Design review of the part built by this model. Coordinates are the model's own, in mm. Face numbers are marked on the shaded views. Coordinates: 2 decimals unless noted, no trailing zeros. Loops run counter-clockwise (first coordinate to the right, second up) from the corner with the lowest first, then second, coordinate; pieces in that order, holes last. Notation, with made-up numbers: (7, 64) - (58, 64) arc R35 cw to (58, 99) - close; hole circle Ø3 at (48, -7). An arc over 180 degrees is marked (long way). Use one line per item in the form item = value. Start each with the question number.
(1) For L1, parallel to Y at x = 4, z = 14; L2, parallel to X at y = 6.5, z = -1.5; L3, parallel to Z at x = 0, y = 16.75, list the stretches that pass through material, from the lowest coordinate up.
(2) Add section B-B (z = 0). State the section outline as (x, y) points.
(3) Clearance check with flat-ended pins moving along their axes: pin 1 Ø1.5 at (y, z) = (15.5, 0.5) entering from -X; pin 2 Ø10 at (x, y) = (2.5, 1) entering from +Z; pin 3 Ø8 at (x, y) = (-4.5, 1) entering from -Z; pin 4 Ø2 at (y, z) = (2, 8) entering from -X. State where each tip first meets the part, or that it passes through.
(4) The part is to be moulded in two halves that separate along X. For the marked faces 1, 2, 3 and 4, say which applies: pulls with the +X half, pulls with the -X half, needs draft (parallel to the pull), parting line crosses it, or undercut.
(5) Add section C-C (x = 6.5). State the section outline as (y, z) points, plus the area to 3 significant figures.
(6) Add section A-A (x = 0). State the section outline as (y, z) points, plus the area to 4 significant figures.
(7) Add section D-D (z = -12.5). State the section outline as (x, y) points, plus the area to 3 significant figures.
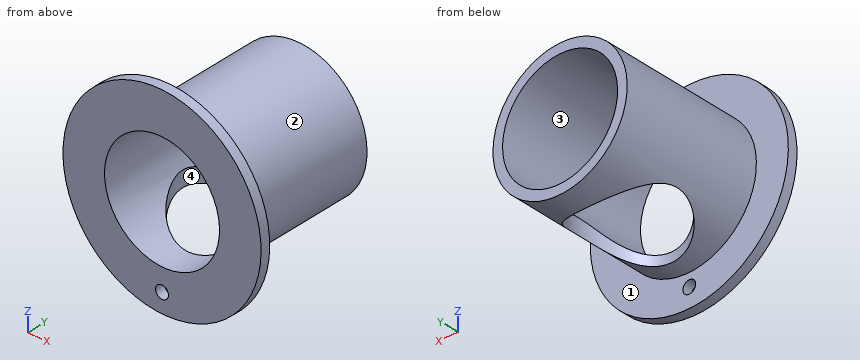
```python
from build123d import *

# Parameters (mm, degrees)
SKETCH1_R           = 10.5
SKETCH1_R_2         = 9
BOSS_EXTRUDE1_DEPTH = 38.3
SKETCH2_R           = 15.5
SKETCH2_R_2         = 9
SKETCH2_R_3         = 1
BOSS_EXTRUDE2_DEPTH = 1.5
SKETCH10_R          = 7.65
CUT_EXTRUDE1_DEPTH  = 46.437209421
SKETCH15_R          = 20.755300819
CUT_EXTRUDE3_DEPTH  = 17.5


with BuildPart() as part:
    # Sketch1 → Boss-Extrude1 (new body)
    with BuildSketch(Plane(origin=(0, 0, 0), x_dir=(1, 0, 0), z_dir=(0, 1, 0))):
        with Locations(Location((0, 0, 0), (0, 0, 270))):
            Circle(SKETCH1_R)
        with Locations(Location((0, 0, 0), (0, 0, 270))):
            Circle(SKETCH1_R_2, mode=Mode.SUBTRACT)
    extrude(amount=BOSS_EXTRUDE1_DEPTH)

    # Sketch2 → Boss-Extrude2 (add)
    with BuildSketch(Plane(origin=(0, 38.3, 0), x_dir=(1, 0, 0), z_dir=(0, 1, 0))):
        with Locations(Location((0, 0, 0), (0, 0, 270))):
            Circle(SKETCH2_R)
        with Locations(Location((0, 0, 0), (0, 0, 270))):
            Circle(SKETCH2_R_2, mode=Mode.SUBTRACT)
        with Locations(Location((0, 12.5, 0), (0, 0, 270))):
            Circle(SKETCH2_R_3, mode=Mode.SUBTRACT)
    boss_extrude2 = extrude(amount=BOSS_EXTRUDE2_DEPTH)

    # Mirror1: Boss-Extrude2 across plane
    add(boss_extrude2.mirror(Plane(origin=(0, 19.15, 0), x_dir=(0, 0, 1), z_dir=(0, -1, 0))))

    # Sketch10 → Cut-Extrude1 (cut, through all)
    with BuildSketch(Plane.XY):
        with Locations(Location((0, 10.55, 0), (0, 0, 90))):
            Circle(SKETCH10_R)
    extrude(amount=-CUT_EXTRUDE1_DEPTH, mode=Mode.SUBTRACT)

    # Sketch15 → Cut-Extrude3 (cut)
    with BuildSketch(Plane(origin=(0, 39.8, 0), x_dir=(1, 0, 0), z_dir=(0, 1, 0))):
        Circle(SKETCH15_R)
    extrude(amount=-CUT_EXTRUDE3_DEPTH, mode=Mode.SUBTRACT)


solid = part.part
```
Computed values:
q1.L1 = -1.5 to 0
q1.L2 = -10.39 to -8.87, 8.87 to 10.39
q1.L3 = 9 to 10.5
q2.outline = (-15.5, -1.5) - (-9, -1.5) - (-9, 22.3) - (-10.5, 22.3) - (-10.5, 0) - (-15.5, 0) - close; (9, -1.5) - (15.5, -1.5) - (15.5, 0) - (10.5, 0) - (10.5, 22.3) - (9, 22.3) - close
q3.pin_1 = -10.5
q3.pin_2 = 15.5
q3.pin_3 = -15.49
q3.pin_4 = -7.83
q4.face_1 = needs draft
q4.face_2 = parting line crosses it
q4.face_3 = undercut
q4.face_4 = undercut
q5.outline = (-1.5, -14.07) - (0, -14.07) - (0, -8.25) - (6.52, -8.25) - (6.52, -6.22) - (-1.5, -6.22) - close; (-1.5, 6.22) - (22.3, 6.22) - (22.3, 8.25) - (0, 8.25) - (0, 14.07) - (-1.5, 14.07) - close; (14.58, -8.25) - (22.3, -8.25) - (22.3, -6.22) - (14.58, -6.22) - close
q5.area = 97.4 mm^2
q6.outline = (-1.5, -15.5) - (0, -15.5) - (0, -13.5) - (-1.5, -13.5) - close; (-1.5, -11.5) - (0, -11.5) - (0, -10.5) - (2.9, -10.5) - (2.9, -9) - (-1.5, -9) - close; (-1.5, 9) - (22.3, 9) - (22.3, 10.5) - (0, 10.5) - (0, 15.5) - (-1.5, 15.5) - close; (18.2, -10.5) - (22.3, -10.5) - (22.3, -9) - (18.2, -9) - close
q6.area = 60.45 mm^2
q7.outline = (-9.17, -1.5) - (-1, -1.5) - (-1, 0) - (-9.17, 0) - close; (1, -1.5) - (9.17, -1.5) - (9.17, 0) - (1, 0) - close
q7.area = 24.5 mm^2
